Autodesk Inventor part; units mm, degrees
ref_plane "YZ Plane" through (0, 0, 0) normal (1, 0, 0) x (0, 1, 0)
ref_plane "XZ Plane" through (0, 0, 0) normal (0, 1, 0) x (-1, 0, 0)
ref_plane "XY Plane" through (0, 0, 0) normal (0, 0, 1) x (1, 0, 0)
sketch "Sketch1" plane through (0, 0, 0) normal (0, 0, 1) x (1, 0, 0)
  line L0 (5, 0) -> (37.3, 0)
  line L1 (42.3, 5) -> (42.3, 37.3)
  line L2 (37.3, 42.3) -> (5, 42.3)
  line L3 (0, 37.3) -> (0, 5)
  arc A0 (5, 42.3) -> (0, 37.3) centre (5, 37.3) ccw
  arc A1 (42.3, 37.3) -> (37.3, 42.3) centre (37.3, 37.3) ccw
  arc A2 (37.3, 0) -> (42.3, 5) centre (37.3, 5) ccw
  arc A3 (0, 5) -> (5, 0) centre (5, 5) ccw
  point P0 (0, 0)
  dimension "d0" = 42.3
  dimension "d1" = 42.3
  dimension "d2" = 5
extrude "Extrusion1" add sketch "Sketch1" along normal blind 43
sketch "Sketch2" plane through (0, 0, 43) normal (0, 0, 1) x (1, 0, 0)
  line L0 (0, 37.3) -> (0, 5)
  line L1 (5, 0) -> (37.3, 0)
  line L2 (37.3, 42.3) -> (5, 42.3)
  circle A0 centre (5.65, 36.65) radius 1.5
  circle A1 centre (36.65, 36.65) radius 1.5
  circle A2 centre (36.65, 5.65) radius 1.5
  circle A3 centre (5.65, 5.65) radius 1.5
  line L3 (5.65, 5.65) -> (21.15, 21.15)
  line L4 (36.65, 5.65) -> (21.15, 21.15)
  line L5 (21.15, 21.15) -> (36.65, 36.65)
  line L6 (21.15, 21.15) -> (5.65, 36.65)
  line L7 (5.65, 36.65) -> (36.65, 36.65)
  line L8 (5.65, 36.65) -> (5.65, 5.65)
  line L9 (21.15, 21.15) -> (21.15, 0)
  line L10 (0, 21.15) -> (21.15, 21.15)
  point P0 (0, 0)
  dimension "d5" = 31
  dimension "d8" = 3
  dimension "d10" = 21.15
  dimension "d11" = 21.15
extrude "Extrusion2" cut sketch "Sketch2" against normal blind 15 contours L7 L8 A0 | A0 L6 L7 | A2 | L8 L6 A0 | L7 L5 A1 | A1 L5 L7 | L8 L3 A3 | A3 L3 L8
sketch "Sketch3" plane through (0, 0, 43) normal (0, 0, 1) x (1, 0, 0)
  line L0 (0, 37.3) -> (0, 5)
  line L1 (5, 0) -> (37.3, 0)
  line L2 (37.3, 42.3) -> (5, 42.3)
  circle A0 centre (21.15, 21.15) radius 11
  line L3 (0, 21.15) -> (21.15, 21.15)
  line L4 (21.15, 21.15) -> (21.15, 0)
  point P0 (0, 0)
  dimension "d14" = 22
extrude "Extrusion3" add sketch "Sketch3" along normal blind 2
sketch "Sketch4" plane through (21.15, 21.15, 45) normal (0, 0, 1) x (1, 0, 0)
  circle A0 centre (0, 0) radius 11
  circle A1 centre (0, 0) radius 2.5
  point P0 (-21.15, -21.15)
  dimension "d19" = 5
extrude "Extrusion4" add sketch "Sketch4" along normal blind 22 contours A1
equation "\"d1\" = d0"
equation "\"d10\" = d11"
properties part number "NEMA17"
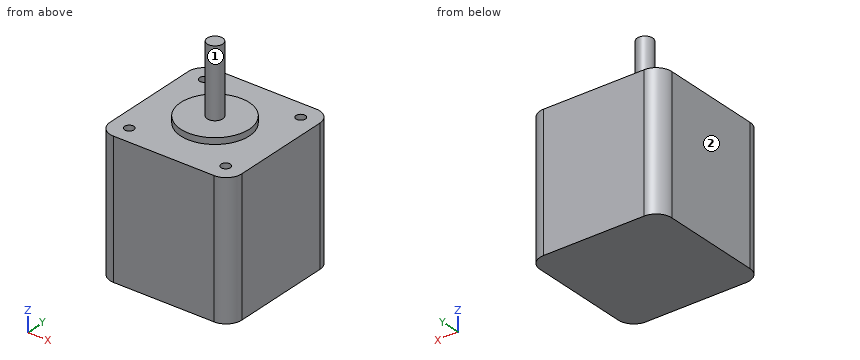
Geometry: final body of the model. Coordinates: model frame, mm. Face numbers are marked on the shaded views. A direction names the side the tool comes from. Give positions to 0.01 mm unless a question says otherwise; leave off trailing zeros. Loops run counter-clockwise (first coordinate to the right, second up) from the corner with the lowest first, then second, coordinate; pieces in that order, holes last. Notation, with made-up numbers: M 39,2 L 97,2 A32 ccw 97,34 Z; hole C 78.25,89.25 d8. An arc over 180 degrees is marked long. Put each result on its own line as item: value. Start each with the question number.
1) Cut plane D-D (z = 53). Output: boundary loops of the cut face in (x, y).
2) Contact query for flat-ended pins moving along their axis: pin 1 (1.5 mm diameter, centred on x = 31, z = 47, fed in from -Y); pin 2 (1.5 mm diameter, centred on x = 36.5, y = 36, fed in from +Z); pin 3 (4 mm diameter, centred on x = 5.65, y = 36.65, fed in from -Z); pin 4 (2 mm diameter, centred on x = 22.5, y = 35.5, fed in from +Z). Output: stop coordinate, or through.
3) Ray query, line 1 along Y through (x, z) = (36.65, 31.25); line 2 along Y through (x, z) = (36, 39). Return the intervals inside material, ascending.
4) Cut plane B-B (x = 21.15). Output: boundary loops of the cut face in (y, z).
5) Cut plane A-A (z = 29). Output: boundary loops of the cut face in (x, y).
6) Access query for the marked faces 1 and 2. Directions: +Z, -Z, +X, -X, +Y, -Y. A direction counts if a zero-diameter tool reaches every point of the face in a straight line with its end or side. Return the directions, or none.
Verdict:
1. outline: C 21.15,21.15 d5
2. pin 1: through
2. pin 2: z = 28
2. pin 3: z = 0
2. pin 4: z = 43
3. line 1: 0 to 4.15, 7.15 to 35.15, 38.15 to 42.3
3. line 2: 0 to 4.3, 7 to 35.3, 38 to 42.3
4. outline: M 0,0 L 42.3,0 L 42.3,43 L 32.15,43 L 32.15,45 L 23.65,45 L 23.65,67 L 18.65,67 L 18.65,45 L 10.15,45 L 10.15,43 L 0,43 Z
5. outline: M 0,5 A5 ccw 5,0 L 37.3,0 A5 ccw 42.3,5 L 42.3,37.3 A5 ccw 37.3,42.3 L 5,42.3 A5 ccw 0,37.3 Z; hole C 5.65,5.65 d3; hole C 5.65,36.65 d3; hole C 36.65,5.65 d3; hole C 36.65,36.65 d3
6. face 1: +Z
6. face 2: +Z, -Z, -X, +Y, -Y
